Drawing for the job (mm, zero at the part's lowest x, y, z). A direction names the side the tool comes from. Coordinates: 2 decimals unless noted, no trailing zeros. Loops run counter-clockwise (first coordinate to the right, second up) from the corner with the lowest first, then second, coordinate; pieces in that order, holes last. Notation, with made-up numbers: (75, 64) -> (109, 64) arc R20 ccw to (109, 73) -> close; hole circle Ø10 at (85.5, 9.25). An arc over 180 degrees is marked (long way). Write item = value, one per line. Start each with the question number.
(1) Drill centre lines: line 1 (X direction, y = 60.5, z = 5.75); line 2 (X direction, y = 20.5, z = 3); line 3 (Z direction, x = 8.5, y = 6). Where is each one in solid material? Low to high. Write a range as from..to.
(2) Band-saw the part on C-C (x = 10). Write the cut outline in (y, z), and give its area (3 significant figures).
(3) Tool access for the marked faces 1, 2 and 3: list every direction of +Z, -Z, +X, -X, +Y, -Y with a clear straight run to the whole face (end or side of a thin tool).
(4) Band-saw the part on B-B (z = 6). Write the cut outline in (x, y).
(5) Band-saw the part on A-A (y = 6). Write the cut outline in (x, z), and give its area (3 significant figures).
(6) Flat gauge pins, fed straight in: P1, Ø3.5, axis at y = 76, z = 5.5, coming from the -X side; P2, Ø6, axis at x = 25.5, z = 5.5, coming from the -Y side; P3, Ø7, axis at y = 6, z = 6, coming from the +X side; P4, Ø8, axis at x = 24.5, y = 49, coming from the -Z side. Where does each tip first touch, or does it go through?
(7) Band-saw the part on D-D (y = 47). Write the cut outline in (x, z).
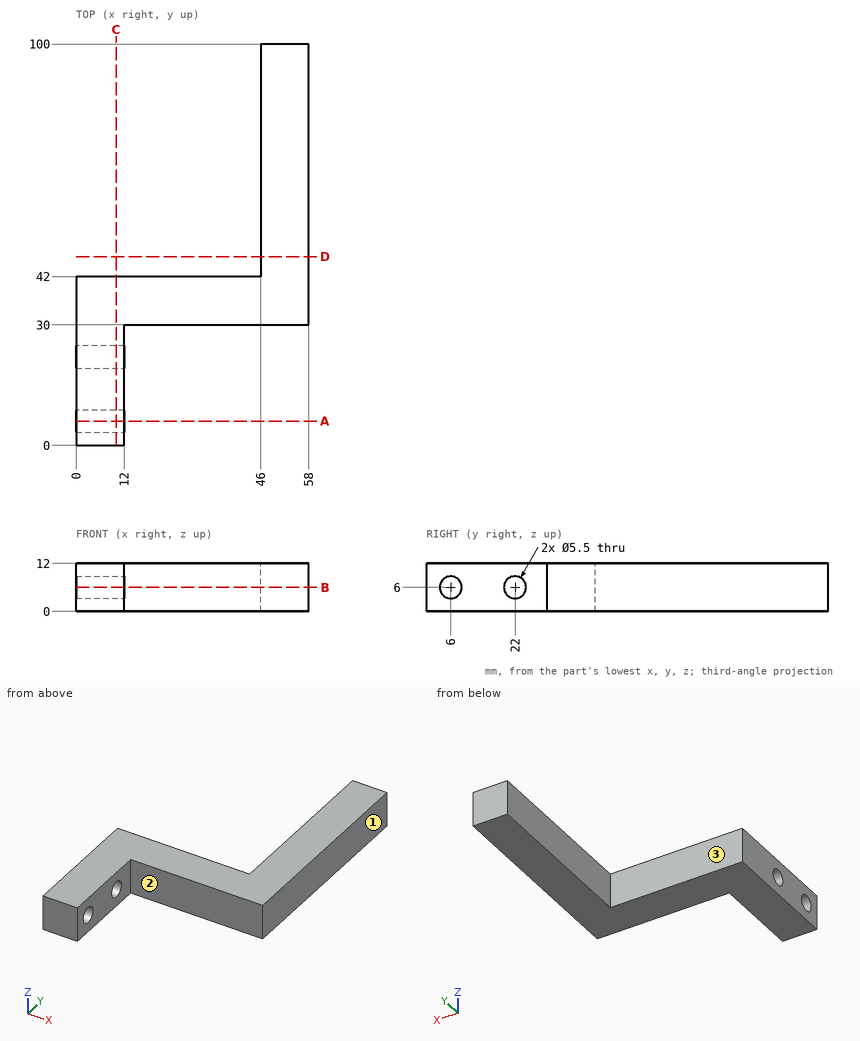
Findings below:
q1.line_1 = 46..58
q1.line_2 = 0..12
q1.line_3 = 0..3.25, 8.75..12
q2.outline = (0, 0) -> (42, 0) -> (42, 12) -> (0, 12) -> close; hole circle Ø5.5 at (6, 6); hole circle Ø5.5 at (22, 6)
q2.area = 456 mm²
q3.face_1 = +Z, -Z, +X, +Y, -Y
q3.face_2 = +Z, -Z, +X, -Y
q3.face_3 = +Z, -Z, -X, +Y
q4.outline = (0, 0) -> (12, 0) -> (12, 3.25) -> (0, 3.25) -> close; (0, 8.75) -> (12, 8.75) -> (12, 19.25) -> (0, 19.25) -> close; (0, 24.75) -> (12, 24.75) -> (12, 30) -> (58, 30) -> (58, 100) -> (46, 100) -> (46, 42) -> (0, 42) -> close
q5.outline = (0, 0) -> (12, 0) -> (12, 3.25) -> (0, 3.25) -> close; (0, 8.75) -> (12, 8.75) -> (12, 12) -> (0, 12) -> close
q5.area = 78.0 mm²
q6.P1 = 46
q6.P2 = 30
q6.P3 = 12
q6.P4 = through
q7.outline = (46, 0) -> (58, 0) -> (58, 12) -> (46, 12) -> close
